from build123d import *

# Parameters (mm, degrees)
CUT_EXTRUDE3_DEPTH           = 60
CUT_EXTRUDE5_DEPTH           = 2
CUT_EXTRUDE5_DEPTH_BACK      = 30
SKETCH9_R                    = 38
SKETCH9_R_2                  = 23
SKETCH19_W                   = 12
SKETCH19_H                   = 36.5
CUT_REVOLVE2_ANGLE           = 65
CUT_REVOLVE2_OTHER_WAY_ANGLE = 65
SKETCH21_W                   = 3.25
SKETCH21_H                   = 4
BOSS_EXTRUDE3_DEPTH          = 1.35
CIRPATTERN1_COUNT            = 5
CUT_EXTRUDE9_START           = -5
CUT_EXTRUDE9_DEPTH           = 5
SKETCH23_R                   = 10.5
CUT_EXTRUDE10_DEPTH          = 10
SKETCH24_W                   = 17
SKETCH24_H                   = 12
BOSS_EXTRUDE4_DEPTH          = 8
SKETCH26_W                   = 12
SKETCH26_H                   = 8
CUT_EXTRUDE11_DEPTH          = 10
SKETCH27_W                   = 4
SKETCH27_H                   = 5
CUT_EXTRUDE12_DEPTH          = 5
CUT_EXTRUDE14_DEPTH          = 2
CUT_EXTRUDE14_DEPTH_BACK     = 30
SKETCH29_R                   = 1
CUT_EXTRUDE15_DEPTH          = 15
FILLET1_R                    = 6
FILLET2_R                    = 8
SKETCH30_W                   = 97.703590575
SKETCH30_H                   = 5
CUT_EXTRUDE16_DEPTH          = 5
INTERSECT1_START             = 20.469057744
INTERSECT1_DEPTH             = 42.958818353


# Read off the part's stored shape, not the designer's step: Cut-Extrude9, Intersect1
with BuildPart() as part:
    # Sketch1 → Revolve1 (revolve)
    with BuildSketch(Plane.XY, mode=Mode.PRIVATE) as revolve1_sk:
        with BuildLine():
            Line((0, 63.427876097), (32, 63.427876097))
            ThreePointArc((32, 63.427876097), (37.656854249, 61.084730346), (40, 55.427876097))
            Line((40, 55.427876097), (40, 28.846818009))
            ThreePointArc((40, 28.846818009), (38.792081772, 24.082439968), (35.460140376, 20.469057744))
            Line((35.460140376, 20.469057744), (28.539859624, 15.958818353))
            ThreePointArc((28.539859624, 15.958818353), (25.207918228, 12.345436129), (24, 7.581058088))
            Line((24, 7.581058088), (24, 3.25))
            Line((24, 3.25), (24.35, 3))
            Line((24.35, 3), (24.35, 0))
            Line((24.35, 0), (22.5, 0))
            Line((22.5, 0), (22.5, 12.5))
            ThreePointArc((22.5, 12.5), (22.353553391, 12.853553391), (22, 13))
            Line((22, 13), (0, 13))
            Line((0, 13), (0, 63.427876097))
        make_face()
    revolve(revolve1_sk.sketch.rotate(Axis((0, 0, 0), (0, 1, 0)), 90), axis=Axis((0, 0, 0), (0, 1, 0)))

    # Sketch11 → Cut-Extrude3 (cut)
    with BuildSketch(Plane(origin=(0, 13, 0), x_dir=(-1, 0, 0), z_dir=(0, -1, 0))):
        with BuildLine():
            Line((-21, 0), (21, 0))
            ThreePointArc((21, 0), (0, 21), (-21, 0))
        make_face()
    extrude(amount=-CUT_EXTRUDE3_DEPTH, mode=Mode.SUBTRACT)

    # Sketch9 → Cut-Extrude5 (cut, two sides: drawn at the far end of the back side and taken through both)
    with BuildSketch(Plane(origin=(0, 55.427876097, 0), x_dir=(1, 0, 0), z_dir=(0, 1, 0)).offset(-CUT_EXTRUDE5_DEPTH_BACK)):
        with Locations(Location((0, 0, 0), (0, 0, 270))):
            Circle(SKETCH9_R)
        with Locations(Location((0, 0, 0), (0, 0, 270))):
            Circle(SKETCH9_R_2, mode=Mode.SUBTRACT)
    extrude(amount=CUT_EXTRUDE5_DEPTH + CUT_EXTRUDE5_DEPTH_BACK, mode=Mode.SUBTRACT)

    # Sketch19 → Cut-Revolve2 (revolve, cut)
    with BuildSketch(Plane(origin=(0, 0, 0), x_dir=(0, 0, -1), z_dir=(1, 0, 0))):
        with Locations((-41.064715832, 37.177876097)):
            Rectangle(SKETCH19_W, SKETCH19_H)
    revolve(axis=Axis((0, 0, 0), (0, 1, 0)), revolution_arc=CUT_REVOLVE2_ANGLE, mode=Mode.SUBTRACT)

    # Sketch19 → Cut-Revolve2 other way (revolve, cut)
    with BuildSketch(Plane(origin=(0, 0, 0), x_dir=(0, 0, -1), z_dir=(1, 0, 0))):
        with Locations((-41.064715832, 37.177876097)):
            Rectangle(SKETCH19_W, SKETCH19_H)
    revolve(axis=Axis((0, 0, 0), (0, -1, 0)), revolution_arc=CUT_REVOLVE2_OTHER_WAY_ANGLE, mode=Mode.SUBTRACT)

    # Sketch21 → Boss-Extrude3 (add)
    with BuildSketch(Plane(origin=(0, 0, 22.5), x_dir=(-1, 0, 0), z_dir=(0, 0, -1))):
        with Locations((0, 2)):
            Rectangle(SKETCH21_W, SKETCH21_H)
    boss_extrude3 = extrude(amount=BOSS_EXTRUDE3_DEPTH)

    # CirPattern1: Boss-Extrude3 ×5 about axis
    cirpattern1_axis = Axis((0, 0, 0), (0, 1, 0))
    for i in range(1, CIRPATTERN1_COUNT):
        add(boss_extrude3.rotate(cirpattern1_axis, i * 360 / CIRPATTERN1_COUNT))

    # Cut-Extrude9 outline → Cut-Extrude9 (cut)
    with BuildSketch(Plane(origin=(0, 63.427876097, 0), x_dir=(1, 0, 0), z_dir=(0, 1, 0)).offset(CUT_EXTRUDE9_START)):
        with BuildLine():
            ThreePointArc((40, 0), (0, 40), (-40, 0))
            Line((-40, 0), (-21, 0))
            ThreePointArc((-21, 0), (0, 21), (21, 0))
            Line((21, 0), (40, 0))
        make_face()
    extrude(amount=CUT_EXTRUDE9_DEPTH, mode=Mode.SUBTRACT)

    # Sketch23 → Cut-Extrude10 (cut)
    with BuildSketch(Plane(origin=(0, 0, -40), x_dir=(-1, 0, 0), z_dir=(0, 0, -1))):
        with Locations((0, 42.137876097)):
            Circle(SKETCH23_R)
    extrude(amount=-CUT_EXTRUDE10_DEPTH, mode=Mode.SUBTRACT)

    # Sketch24 → Boss-Extrude4 (add)
    with BuildSketch(Plane(origin=(0, 58.427876097, 0), x_dir=(1, 0, 0), z_dir=(0, 1, 0))):
        with Locations((0, 30)):
            Rectangle(SKETCH24_W, SKETCH24_H)
    extrude(amount=-BOSS_EXTRUDE4_DEPTH)

    # Sketch26 → Cut-Extrude11 (cut)
    with BuildSketch(Plane(origin=(0, 58.427876097, 0), x_dir=(1, 0, 0), z_dir=(0, 1, 0))):
        with Locations((0, 30)):
            Rectangle(SKETCH26_W, SKETCH26_H)
    extrude(amount=-CUT_EXTRUDE11_DEPTH, mode=Mode.SUBTRACT)

    # Sketch27 → Cut-Extrude12 (cut)
    with BuildSketch(Plane(origin=(8.5, 0, 0), x_dir=(0, 0, -1), z_dir=(1, 0, 0))):
        with Locations((29.5, 53.927876097)):
            Rectangle(SKETCH27_W, SKETCH27_H)
    extrude(amount=-CUT_EXTRUDE12_DEPTH, mode=Mode.SUBTRACT)

    # Sketch28 → Cut-Extrude14 (cut, two sides: drawn at the far end of the back side and taken through both)
    with BuildSketch(Plane(origin=(0, 55.427876097, 0), x_dir=(1, 0, 0), z_dir=(0, 1, 0)).offset(-CUT_EXTRUDE14_DEPTH_BACK)):
        with BuildLine():
            Line((-22.912878475, -2), (22.912878475, -2))
            ThreePointArc((22.912878475, -2), (0, -23), (-22.912878475, -2))
        make_face()
    extrude(amount=CUT_EXTRUDE14_DEPTH + CUT_EXTRUDE14_DEPTH_BACK, mode=Mode.SUBTRACT)

    # Sketch29 → Cut-Extrude15 (cut)
    with BuildSketch(Plane(origin=(0, 0, 0), x_dir=(-1, 0, 0), z_dir=(0, 0, -1))):
        with Locations((-30.416198487, 60.927876097)):
            Circle(SKETCH29_R)
        with Locations((30.416198487, 60.927876097)):
            Circle(SKETCH29_R)
        with Locations((0, 60.927876097)):
            Circle(SKETCH29_R)
    extrude(amount=-CUT_EXTRUDE15_DEPTH, mode=Mode.SUBTRACT)

    # Fillet1
    fillet1_edges = [part.edges().sort_by_distance(p)[0] for p in [
        (21, 35.713938048, 0),
        (-21, 35.713938048, 0),
    ]]
    fillet(fillet1_edges, radius=FILLET1_R)

    # Fillet2
    fillet2_edges = [part.edges().sort_by_distance(p)[0] for p in [
        (-22.912878475, 41.427876097, 2),
        (22.912878475, 41.427876097, 2),
    ]]
    fillet(fillet2_edges, radius=FILLET2_R)

    # Sketch30 → Cut-Extrude16 (cut)
    with BuildSketch(Plane(origin=(0, 63.427876097, 0), x_dir=(1, 0, 0), z_dir=(0, 1, 0))):
        with Locations((-0.528699084, -2.5)):
            Rectangle(SKETCH30_W, SKETCH30_H)
    extrude(amount=-CUT_EXTRUDE16_DEPTH, mode=Mode.SUBTRACT)

    # Intersect1 outline → Intersect1 (cut)
    with BuildSketch(Plane(origin=(0, 0, 0), x_dir=(1, 0, 0), z_dir=(0, 1, 0)).offset(INTERSECT1_START)):
        with BuildLine():
            Line((-37.080992435, -15), (-42, -15))
            Line((-42, -15), (-42, -42))
            Line((-42, -42), (42, -42))
            Line((42, -42), (42, -15))
            Line((42, -15), (37.080992435, -15))
            ThreePointArc((37.080992435, -15), (0, 40), (-37.080992435, -15))
        make_face()
        with BuildLine():
            Line((13.747727085, 0), (-13.747727085, 0))
            ThreePointArc((-13.747727085, 0), (-18.767687244, 2.713664655), (-19.246817919, 8.4))
            ThreePointArc((-19.246817919, 8.4), (0, 21), (19.246817919, 8.4))
            ThreePointArc((19.246817919, 8.4), (18.767687244, 2.713664655), (13.747727085, 0))
        make_face(mode=Mode.SUBTRACT)
    extrude(amount=INTERSECT1_DEPTH, mode=Mode.SUBTRACT)


solid = part.part
Source: CAD feature listing. Evaluate the final solid. Frame: model axes, mm. A direction names the side the tool comes from. Round coordinates to 2 decimals unless told otherwise and drop trailing zeros. Write each loop counter-clockwise with the first axis right and the second up, starting at its lowest first coordinate (ties: lowest second). Pieces come first, ordered by that corner, then holes. Notation, with made-up numbers: M 12,84.5 L 52,84.5 A8 ccw 52,89.5 Z; hole C 77.5,41.5 d1. An arc over 180 degrees is marked long. One line per item, written item: value. Start each with the question number.
Item 1: Mould query, pull axis Y, two halves, no side actions, for faces 1 (the conical face through (25.62, 16.18, -13.32)), 2 (the flat face through (-20.108, 2.028, 6.557)), 3 (the flat face through (-13, 4, -18)). Classes: pulls with the +Y half, pulls with the -Y half, needs draft (parallel to the pull), parting line crosses it, or undercut.
Item 2: Section query B-B (y = 14.25). Return the cut outline in (x, z), plus the area to 3 significant figures.
Item 3: Section query A-A (x = 0). Return the cut outline in (y, z), plus the area to 3 significant figures.
Item 4: Pin query (flat end, axial travel): pin 1 (1 mm diameter, centred on y = 8.5, z = -14.5, fed in from -X); pin 2 (8 mm diameter, centred on x = 23.5, y = 6, fed in from -Z); pin 3 (3 mm diameter, centred on y = 17, z = -21.5, fed in from +X); pin 4 (12 mm diameter, centred on x = 15, z = 4, fed in from -Y). Return the tip coordinate at first contact, or that it passes through.
Item 5: Set-up query: faces 4 (the flat face through (0, 20.469, 7)), 5 (the cylindrical face through (-7.21, 5.39, -22.89)), 6 (the cylindrical face through (14.82, 1.48, 19.32)), 7 (the cylindrical face through (0, 17, -21)). Return all of +Z, -Z, +X, -X, +Y, -Y with unobstructed straight access to the full face (end or side cutting, diameter ignored); none if empty.
Item 6: Ray query, L1, parallel to X at y = 7.25, z = 0; L2, parallel to Y at x = 15.5, z = 6.5; L3, parallel to Z at x = 20.5, y = 12. Return the intervals inside material, ascending. Write a range as from..to.
Result set:
1. face 1: pulls with the -Y half
1. face 2: needs draft
1. face 3: undercut
2. outline: C 0,0 d53.1; hole M -19.25,-8.4 A21 ccw 19.25,-8.4 A6 ccw 13.75,0 L -13.75,0 A6 ccw Z
2. area: 1,550 mm²
3. outline: M 0,-24.35 L 3,-24.35 L 3.25,-24 L 7.58,-24 A10 cw 15.96,-28.54 L 20.47,-35.46 L 20.47,-21 L 13,-21 L 13,-22 A0.5 cw 12.5,-22.5 L 0,-22.5 Z; M 0,21.15 L 4,21.15 L 4,22.5 L 12.5,22.5 A0.5 cw 13,22 L 13,0 L 20.47,0 L 20.47,35.06 L 20.21,35.06 L 15.96,28.54 A10 cw 7.58,24 L 3.25,24 L 3,24.35 L 0,24.35 Z
3. area: 343 mm²
4. pin 1: stops at x = -19.55
4. pin 2: stops at z = -13.99
4. pin 3: stops at x = 24.56
4. pin 4: stops at y = 0
5. face 4: +Z, -Z, +X, -X, +Y
5. face 5: none
5. face 6: -Y
5. face 7: +Y, -Y
6. L1: x = -24..-22.5, 22.5..24
6. L2: y = 13..20.47
6. L3: z = -14.36..-9.27, 9.27..14.36
